Can you work these out from the model? Positions are in its coordinate system, mm. Face numbers are marked on the shaded views. A direction names the side the tool comes from. Round coordinates to 2 decimals unless told otherwise and drop trailing zeros. Loops run counter-clockwise (first coordinate to the right, second up) from the corner with the lowest first, then second, coordinate; pieces in that order, holes last.
(1) I want a section at A-A on z = 9.5. Write out the boundary of the cut face in (x, y), plus the area to 3 significant figures.
(2) Will these pins go through, and if not, where does the flat tip stop? pin 1 Ø2 at (x, z) = (5, 13.5) entering from +Y; pin 2 Ø5.5 at (x, z) = (4.2, 30) entering from +Y.
(3) If I drill on line 1 along Z through (x, y) = (4.2, 2.8); line 2 along Z through (x, y) = (23.8, 1.85); line 3 along X through (y, z) = (2.55, 55), over which ranges is the centre line in solid material (lowest first)?
(4) Which directions (+Z, -Z, +X, -X, +Y, -Y) give clear straight access to the entire face, cutting with the end or side of a thin tool? Please do the marked faces 3 and 4.
(5) I want a section at B-B on z = 50. Write out the boundary of the cut face in (x, y).
(6) Thinking about a two-plate mould opening in X: for the marked faces 1 and 2, which applies, released by +X, released by -X, zero draft, split by the parting line, or undercut?
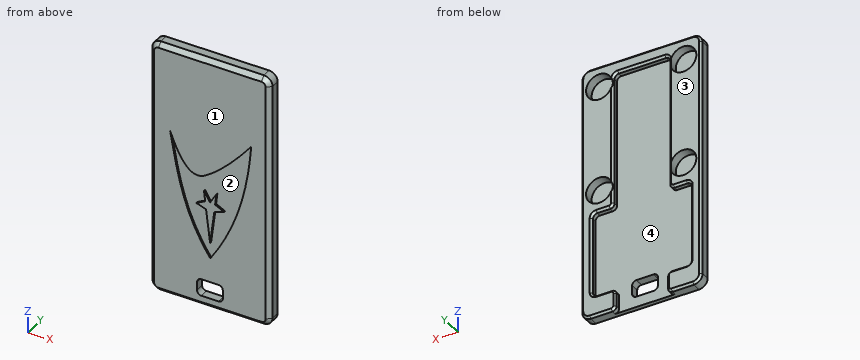
from build123d import *

# Parameters (mm, degrees)
SKETCH1_R           = 3.05
BOSS_EXTRUDE1_DEPTH = 3.5
SKETCH1_3_W         = 13
SKETCH1_3_H         = 32
SKETCH1_3_W_2       = 12
SKETCH1_3_H_2       = 5
BOSS_EXTRUDE2_DEPTH = 2
SKETCH1_4_R         = 3.05
BOSS_EXTRUDE3_DEPTH = 1.3
SKETCH2_W           = 6
SKETCH2_H           = 4
CUT_EXTRUDE1_DEPTH  = 4
FILLET1_R           = 1
FILLET2_R           = 1
FILLET3_R           = 1
FILLET4_R           = 2
CHAMFER1_SIZE       = 1
CHAMFER2_SIZE       = 0.5
CUT_EXTRUDE2_DEPTH  = 0.4


with BuildPart() as part:
    # Sketch1 → Boss-Extrude1 (new body)
    with BuildSketch(Plane(origin=(0, 0, 0), x_dir=(1, 0, 0), z_dir=(0, 1, 0))):
        Polygon((8, 0), (0, 0), (0, -60), (28, -60), (28, 0), (20, 0), (20, -5), (25.5, -5), (25.5, -25), (20.5, -25), (20.5, -57), (7.5, -57), (7.5, -25), (2.5, -25), (2.5, -5), (8, -5), align=None)
        with Locations(Location((4.2, -55, 0), (0, 0, 270))):
            Circle(SKETCH1_R, mode=Mode.SUBTRACT)
        with Locations(Location((4.2, -30, 0), (0, 0, 270))):
            Circle(SKETCH1_R, mode=Mode.SUBTRACT)
        with Locations(Location((23.8, -55, 0), (0, 0, 270))):
            Circle(SKETCH1_R, mode=Mode.SUBTRACT)
        with Locations(Location((23.8, -30, 0), (0, 0, 270))):
            Circle(SKETCH1_R, mode=Mode.SUBTRACT)
    extrude(amount=BOSS_EXTRUDE1_DEPTH)

    # Sketch1<3> → Boss-Extrude2 (add)
    with BuildSketch(Plane(origin=(0, 0, 0), x_dir=(1, 0, 0), z_dir=(0, 1, 0))):
        with Locations((14, -41)):
            Rectangle(SKETCH1_3_W, SKETCH1_3_H)
        Polygon((20, -5), (8, -5), (2.5, -5), (2.5, -25), (7.5, -25), (20.5, -25), (25.5, -25), (25.5, -5), align=None)
        with Locations((14, -2.5)):
            Rectangle(SKETCH1_3_W_2, SKETCH1_3_H_2)
    extrude(amount=BOSS_EXTRUDE2_DEPTH)

    # Sketch1<4> → Boss-Extrude3 (add)
    with BuildSketch(Plane(origin=(0, 0, 0), x_dir=(1, 0, 0), z_dir=(0, 1, 0))):
        with Locations(Location((4.2, -30, 0), (0, 0, 270))):
            Circle(SKETCH1_4_R)
        with Locations(Location((23.8, -30, 0), (0, 0, 270))):
            Circle(SKETCH1_4_R)
        with Locations(Location((4.2, -55, 0), (0, 0, 270))):
            Circle(SKETCH1_4_R)
        with Locations(Location((23.8, -55, 0), (0, 0, 270))):
            Circle(SKETCH1_4_R)
    extrude(amount=BOSS_EXTRUDE3_DEPTH)

    # Sketch2 → Cut-Extrude1 (cut)
    with BuildSketch(Plane(origin=(0, 2, 0), x_dir=(1, 0, 0), z_dir=(0, 1, 0))):
        with Locations((14, -4.5)):
            Rectangle(SKETCH2_W, SKETCH2_H)
    extrude(amount=-CUT_EXTRUDE1_DEPTH, mode=Mode.SUBTRACT)

    # Fillet1
    fillet1_edges = [part.edges().sort_by_distance(p)[0] for p in [
        (11, 1, 6.5),
        (11, 1, 2.5),
        (17, 1, 2.5),
        (17, 1, 6.5),
    ]]
    fillet(fillet1_edges, radius=FILLET1_R)

    # Fillet2
    fillet2_edges = [part.edges().sort_by_distance(p)[0] for p in [
        (25.5, 2.75, 25),
        (25.5, 2.75, 5),
        (20, 2.75, 5),
        (8, 2.75, 5),
        (2.5, 2.75, 5),
        (2.5, 2.75, 25),
        (7.5, 2.75, 25),
        (7.5, 2.75, 57),
        (20.5, 2.75, 57),
        (20.5, 2.75, 25),
    ]]
    fillet(fillet2_edges, radius=FILLET2_R)

    # Fillet3
    fillet3_edges = [part.edges().sort_by_distance(p)[0] for p in [
        (20, 2.75, 0),
        (8, 2.75, 0),
    ]]
    fillet(fillet3_edges, radius=FILLET3_R)

    # Fillet4
    fillet4_edges = [part.edges().sort_by_distance(p)[0] for p in [
        (28, 1.75, 0),
        (28, 1.75, 60),
        (0, 1.75, 60),
        (0, 1.75, 0),
    ]]
    fillet(fillet4_edges, radius=FILLET4_R)

    # Chamfer1
    chamfer1_edges = [part.edges().sort_by_distance(p)[0] for p in [
        (28, 0, 30),
        (0, 0, 30),
        (14, 0, 0),
        (14, 0, 60),
        (0.585786438, 0, 0.585786438),
        (27.414213562, 0, 0.585786438),
        (0.585786438, 0, 59.414213562),
        (27.414213562, 0, 59.414213562),
    ]]
    chamfer(chamfer1_edges, length=CHAMFER1_SIZE)

    # Chamfer2
    # the kernel refuses this chamfer: 0.5 mm, written as the material it takes off along each edge
    with BuildSketch(Plane(origin=(8.5, 3.5, 56), x_dir=(-1, 0, 0), z_dir=(0, 0, -1))) as chamfer2_piece_1:
        Polygon((1 + CHAMFER2_SIZE, 0), (1, -CHAMFER2_SIZE), (1, 0), align=None)
    revolve(axis=Axis((8.5, 3.5, 56), (0, 1, 0)), revolution_arc=90, mode=Mode.SUBTRACT)
    with BuildSketch(Plane(origin=(7.5, 3.5, 56), x_dir=(-0.9996219169112968, 0.02749587661058651, 0), z_dir=(0, 0, -1)), Plane(origin=(20.5, 3.5, 26), x_dir=(0.9996219169112968, 0.027495876610586414, 0), z_dir=(0, 0, 1))) as chamfer2_piece_2:
        Polygon((CHAMFER2_SIZE * 0.999621916911, -CHAMFER2_SIZE * 0.0274958766106), (-CHAMFER2_SIZE * 0.0274958766106, -CHAMFER2_SIZE * 0.999621916911), (0, 0), align=None)
    extrude(amount=30, mode=Mode.SUBTRACT)
    with BuildSketch(Plane(origin=(19.5, 3.5, 57), x_dir=(0, 0.027495876610586605, 0.9996219169112968), z_dir=(-1, 0, 0))) as chamfer2_piece_3:
        Polygon((CHAMFER2_SIZE * 0.999621916911, -CHAMFER2_SIZE * 0.0274958766106), (-CHAMFER2_SIZE * 0.0274958766106, -CHAMFER2_SIZE * 0.999621916911), (0, 0), align=None)
    extrude(amount=11, mode=Mode.SUBTRACT)
    with BuildSketch(Plane(origin=(6.5, 3.5, 26), x_dir=(0, 0, -1), z_dir=(-1, 0, 0))) as chamfer2_piece_4:
        Polygon((1 - CHAMFER2_SIZE, 0), (1, CHAMFER2_SIZE), (1, 0), align=None)
    revolve(axis=Axis((6.5, 3.5, 26), (0, -1, 0)), revolution_arc=90, mode=Mode.SUBTRACT)
    with BuildSketch(Plane(origin=(19.5, 3.5, 56), x_dir=(0, 0, 1), z_dir=(-1, 0, 0))) as chamfer2_piece_5:
        Polygon((1 + CHAMFER2_SIZE, 0), (1, -CHAMFER2_SIZE), (1, 0), align=None)
    revolve(axis=Axis((19.5, 3.5, 56), (0, 1, 0)), revolution_arc=90, mode=Mode.SUBTRACT)
    with BuildSketch(Plane(origin=(6.5, 3.5, 25), x_dir=(0, 0.027495876610586414, 0.9996219169112968), z_dir=(-1, 0, 0)), Plane(origin=(24.5, 3.5, 25), x_dir=(0, 0.027495876610586414, 0.9996219169112968), z_dir=(-1, 0, 0)), Plane(origin=(8, 3.5, 4), x_dir=(-0.9996219169112968, 0.02749587661058651, 0), z_dir=(0, 0, -1)), Plane(origin=(20, 3.5, 1), x_dir=(0.9996219169112968, 0.027495876610586414, 0), z_dir=(0, 0, 1))) as chamfer2_piece_6:
        Polygon((CHAMFER2_SIZE * 0.999621916911, -CHAMFER2_SIZE * 0.0274958766106), (-CHAMFER2_SIZE * 0.0274958766106, -CHAMFER2_SIZE * 0.999621916911), (0, 0), align=None)
    extrude(amount=3, mode=Mode.SUBTRACT)
    with BuildSketch(Plane(origin=(3.5, 3.5, 24), x_dir=(-1, 0, 0), z_dir=(0, 0, -1))) as chamfer2_piece_7:
        Polygon((1 + CHAMFER2_SIZE, 0), (1, -CHAMFER2_SIZE), (1, 0), align=None)
    revolve(axis=Axis((3.5, 3.5, 24), (0, 1, 0)), revolution_arc=90, mode=Mode.SUBTRACT)
    with BuildSketch(Plane(origin=(21.5, 3.5, 26), x_dir=(-1, 0, 0), z_dir=(0, 0, 1))) as chamfer2_piece_8:
        Polygon((1 - CHAMFER2_SIZE, 0), (1, CHAMFER2_SIZE), (1, 0), align=None)
    revolve(axis=Axis((21.5, 3.5, 26), (0, -1, 0)), revolution_arc=90, mode=Mode.SUBTRACT)
    with BuildSketch(Plane(origin=(2.5, 3.5, 24), x_dir=(-0.9996219169112968, 0.027495876610586438, 0), z_dir=(0, 0, -1)), Plane(origin=(25.5, 3.5, 6), x_dir=(0.9996219169112968, 0.027495876610586414, 0), z_dir=(0, 0, 1))) as chamfer2_piece_9:
        Polygon((CHAMFER2_SIZE * 0.999621916911, -CHAMFER2_SIZE * 0.0274958766106), (-CHAMFER2_SIZE * 0.0274958766106, -CHAMFER2_SIZE * 0.999621916911), (0, 0), align=None)
    extrude(amount=18, mode=Mode.SUBTRACT)
    with BuildSketch(Plane(origin=(3.5, 3.5, 6), x_dir=(0, 0, -1), z_dir=(1, 0, 0))) as chamfer2_piece_10:
        Polygon((1 + CHAMFER2_SIZE, 0), (1, -CHAMFER2_SIZE), (1, 0), align=None)
    revolve(axis=Axis((3.5, 3.5, 6), (0, 1, 0)), revolution_arc=90, mode=Mode.SUBTRACT)
    with BuildSketch(Plane(origin=(24.5, 3.5, 24), x_dir=(1, 0, 0), z_dir=(0, 0, -1))) as chamfer2_piece_11:
        Polygon((1 + CHAMFER2_SIZE, 0), (1, CHAMFER2_SIZE), (1, 0), align=None)
    revolve(axis=Axis((24.5, 3.5, 24), (0, -1, 0)), revolution_arc=90, mode=Mode.SUBTRACT)
    with BuildSketch(Plane(origin=(3.5, 3.5, 5), x_dir=(0, 0.02749587661058651, -0.9996219169112968), z_dir=(1, 0, 0)), Plane(origin=(21, 3.5, 5), x_dir=(0, 0.027495876610586414, -0.9996219169112968), z_dir=(1, 0, 0))) as chamfer2_piece_12:
        Polygon((CHAMFER2_SIZE * 0.999621916911, -CHAMFER2_SIZE * 0.0274958766106), (-CHAMFER2_SIZE * 0.0274958766106, -CHAMFER2_SIZE * 0.999621916911), (0, 0), align=None)
    extrude(amount=3.5, mode=Mode.SUBTRACT)
    with BuildSketch(Plane(origin=(7, 3.5, 4), x_dir=(0, 0, 1), z_dir=(-1, 0, 0))) as chamfer2_piece_13:
        Polygon((1 - CHAMFER2_SIZE, 0), (1, -CHAMFER2_SIZE), (1, 0), align=None)
    revolve(axis=Axis((7, 3.5, 4), (0, 1, 0)), revolution_arc=90, mode=Mode.SUBTRACT)
    with BuildSketch(Plane(origin=(24.5, 3.5, 6), x_dir=(0, 0, -1), z_dir=(-1, 0, 0))) as chamfer2_piece_14:
        Polygon((1 + CHAMFER2_SIZE, 0), (1, CHAMFER2_SIZE), (1, 0), align=None)
    revolve(axis=Axis((24.5, 3.5, 6), (0, -1, 0)), revolution_arc=90, mode=Mode.SUBTRACT)
    with BuildSketch(Plane(origin=(7, 3.5, 1), x_dir=(1, 0, 0), z_dir=(0, 0, 1))) as chamfer2_piece_15:
        Polygon((1 - CHAMFER2_SIZE, 0), (1, -CHAMFER2_SIZE), (1, 0), align=None)
    revolve(axis=Axis((7, 3.5, 1), (0, 1, 0)), revolution_arc=90, mode=Mode.SUBTRACT)
    with BuildSketch(Plane(origin=(21, 3.5, 4), x_dir=(-1, 0, 0), z_dir=(0, 0, -1))) as chamfer2_piece_16:
        Polygon((1 - CHAMFER2_SIZE, 0), (1, -CHAMFER2_SIZE), (1, 0), align=None)
    revolve(axis=Axis((21, 3.5, 4), (0, 1, 0)), revolution_arc=90, mode=Mode.SUBTRACT)
    with BuildSketch(Plane(origin=(7, 3.5, 0), x_dir=(0, -0.9996219169112968, -0.027495876610586365), z_dir=(-1, 0, 0)), Plane(origin=(26, 3.5, 0), x_dir=(0, -0.9996219169112968, -0.027495876610586365), z_dir=(-1, 0, 0))) as chamfer2_piece_17:
        Polygon((CHAMFER2_SIZE * 0.999621916911, CHAMFER2_SIZE * 0.0274958766106), (-CHAMFER2_SIZE * 0.0274958766106, CHAMFER2_SIZE * 0.999621916911), (0, 0), align=None)
    extrude(amount=5, mode=Mode.SUBTRACT)
    with BuildSketch(Plane(origin=(2, 3.5, 2), x_dir=(-1, 0, 0), z_dir=(0, 0, 1))) as chamfer2_piece_18:
        Polygon((2, CHAMFER2_SIZE), (2 - CHAMFER2_SIZE, 0), (2, 0), align=None)
    revolve(axis=Axis((2, 3.5, 2), (0, -1, 0)), revolution_arc=90, mode=Mode.SUBTRACT)
    with BuildSketch(Plane(origin=(21, 3.5, 1), x_dir=(0, 0, -1), z_dir=(1, 0, 0))) as chamfer2_piece_19:
        Polygon((1 - CHAMFER2_SIZE, 0), (1, -CHAMFER2_SIZE), (1, 0), align=None)
    revolve(axis=Axis((21, 3.5, 1), (0, 1, 0)), revolution_arc=90, mode=Mode.SUBTRACT)
    with BuildSketch(Plane(origin=(0, 3.5, 2), x_dir=(-0.02749587661058636, -0.9996219169112968, 0), z_dir=(0, 0, 1)), Plane(origin=(28, 3.5, 58), x_dir=(0.02749587661058907, -0.9996219169112965, 0), z_dir=(0, 0, -1))) as chamfer2_piece_20:
        Polygon((CHAMFER2_SIZE * 0.999621916911, CHAMFER2_SIZE * 0.0274958766106), (-CHAMFER2_SIZE * 0.0274958766106, CHAMFER2_SIZE * 0.999621916911), (0, 0), align=None)
    extrude(amount=56, mode=Mode.SUBTRACT)
    with BuildSketch(Plane(origin=(2, 3.5, 58), x_dir=(0, 0, 1), z_dir=(1, 0, 0))) as chamfer2_piece_21:
        Polygon((2, CHAMFER2_SIZE), (2 - CHAMFER2_SIZE, 0), (2, 0), align=None)
    revolve(axis=Axis((2, 3.5, 58), (0, -1, 0)), revolution_arc=90, mode=Mode.SUBTRACT)
    with BuildSketch(Plane(origin=(26, 3.5, 2), x_dir=(1, 0, 0), z_dir=(0, 0, 1))) as chamfer2_piece_22:
        Polygon((2, -CHAMFER2_SIZE), (2 - CHAMFER2_SIZE, 0), (2, 0), align=None)
    revolve(axis=Axis((26, 3.5, 2), (0, 1, 0)), revolution_arc=90, mode=Mode.SUBTRACT)
    with BuildSketch(Plane(origin=(2, 3.5, 60), x_dir=(0, -0.999621916911297, 0.027495876610582174), z_dir=(1, 0, 0))) as chamfer2_piece_23:
        Polygon((CHAMFER2_SIZE * 0.999621916911, CHAMFER2_SIZE * 0.0274958766106), (-CHAMFER2_SIZE * 0.0274958766106, CHAMFER2_SIZE * 0.999621916911), (0, 0), align=None)
    extrude(amount=24, mode=Mode.SUBTRACT)
    with BuildSketch(Plane(origin=(26, 3.5, 58), x_dir=(1, 0, 0), z_dir=(0, 0, -1))) as chamfer2_piece_24:
        Polygon((2, CHAMFER2_SIZE), (2 - CHAMFER2_SIZE, 0), (2, 0), align=None)
    revolve(axis=Axis((26, 3.5, 58), (0, -1, 0)), revolution_arc=90, mode=Mode.SUBTRACT)

    # Sketch3 → Cut-Extrude2 (cut)
    with BuildSketch(Plane.XZ):
        with BuildLine():
            add(Edge.make_bspline(
                [(14.097910653, 12.243532923), (20.639688273, 22.096806587), (22.846088229, 32.130025027), (23.610210653, 42.464770423)],
                knots=[0, 0, 0, 0, 1, 1, 1, 1], degree=3))
            add(Edge.make_bspline(
                [(23.610210653, 42.464770423), (19.368087057, 37.051812999), (15.634224065, 33.503649915), (12.891410653, 31.855507923)],
                knots=[0, 0, 0, 0, 1, 1, 1, 1], degree=3))
            add(Edge.make_bspline(
                [(12.891410653, 31.855507923), (9.863152041, 30.035843795), (7.255065309, 32.914045303), (4.691973153, 40.020020423)],
                knots=[0, 0, 0, 0, 1, 1, 1, 1], degree=3))
            add(Edge.make_bspline(
                [(4.691973153, 40.020020423), (6.392651997, 30.746919843), (7.568627293, 21.672393415), (14.097910653, 12.243532923)],
                knots=[0, 0, 0, 0, 1, 1, 1, 1], degree=3))
        make_face()
        Polygon((14.045523153, 15.977332923), (13.094610653, 23.749732923), (10.805435653, 24.529195423), (12.886648153, 25.634095423), (12.612010653, 28.113770423), (14.020123153, 25.711882923), (15.502848153, 28.204257923), (15.202810653, 25.594407923), (17.320535653, 24.527607923), (15.021835653, 23.765607923), align=None, mode=Mode.SUBTRACT)
    extrude(amount=-CUT_EXTRUDE2_DEPTH, mode=Mode.SUBTRACT)


solid = part.part
Filled sheet:
1. outline: (0, 1) - (1, 0) - (27, 0) - (28, 1) - (28, 3) - (27.5, 3.5) - (26, 3.5) - (25.5, 3) - (25.5, 2) - (2.5, 2) - (2.5, 3) - (2, 3.5) - (0.5, 3.5) - (0, 3) - close
1. area: 62.0 mm2
2. pin 1: stops at y = 2
2. pin 2: stops at y = 1.3
3. line 1: z = 0 to 5, 25 to 26.95, 33.05 to 51.95, 58.05 to 60
3. line 2: z = 0 to 26.95, 33.05 to 51.95, 58.05 to 60
3. line 3: x = 0 to 1.15, 7.25 to 7.5, 20.5 to 20.75, 26.85 to 28
4. face 3: +Z, -Z, +X, -X, +Y
4. face 4: +Y
5. outline: (0, 1) - (1, 0) - (27, 0) - (28, 1) - (28, 3) - (27.5, 3.5) - (21, 3.5) - (20.5, 3) - (20.5, 2) - (7.5, 2) - (7.5, 3) - (7, 3.5) - (0.5, 3.5) - (0, 3) - close
6. face 1: zero draft
6. face 2: undercut
